from build123d import *

# Parameters (mm, degrees)
SKETCH1_W           = 74
SKETCH1_H           = 50
BOSS_EXTRUDE1_DEPTH = 10
SKETCH2_W           = 10
SKETCH2_H           = 50
BOSS_EXTRUDE2_DEPTH = 65
SKETCH3_R           = 5
CUT_EXTRUDE1_DEPTH  = 60
SKETCH4_R           = 5
CUT_EXTRUDE3_DEPTH  = 60


with BuildPart() as part:
    # Sketch1 → Boss-Extrude1 (new body)
    with BuildSketch(Plane(origin=(0, 0, 0), x_dir=(1, 0, 0), z_dir=(0, 1, 0))):
        Rectangle(SKETCH1_W, SKETCH1_H)
    extrude(amount=BOSS_EXTRUDE1_DEPTH)

    # Sketch2 → Boss-Extrude2 (add)
    with BuildSketch(Plane(origin=(0, 10, 0), x_dir=(1, 0, 0), z_dir=(0, 1, 0))):
        with Locations((-32, 0)):
            Rectangle(SKETCH2_W, SKETCH2_H)
        with Locations((32, 0)):
            Rectangle(SKETCH2_W, SKETCH2_H)
    extrude(amount=BOSS_EXTRUDE2_DEPTH)

    # Sketch3 → Cut-Extrude1 (cut)
    with BuildSketch(Plane(origin=(-27, 0, 0), x_dir=(0, 0, -1), z_dir=(1, 0, 0))):
        with Locations((0, 65)):
            Circle(SKETCH3_R)
    extrude(amount=-CUT_EXTRUDE1_DEPTH, mode=Mode.SUBTRACT)

    # Sketch4 → Cut-Extrude3 (cut)
    with BuildSketch(Plane.ZY.offset(-27)):
        with Locations((0, 60)):
            Circle(SKETCH4_R)
    extrude(amount=-CUT_EXTRUDE3_DEPTH, mode=Mode.SUBTRACT)


solid = part.part
Geometry check sheet. Reference: the model listing, model coordinates, mm. A direction names the side the tool comes from. Round coordinates to 2 decimals unless told otherwise and drop trailing zeros. Loops run counter-clockwise (first coordinate to the right, second up) from the corner with the lowest first, then second, coordinate; pieces in that order, holes last. Notation, with made-up numbers: (4.5, 52.25) - (13.5, 52.25) arc R33 cw to (13.5, 84.25) - close; hole circle Ø6 at (75.5, 34.5). An arc over 180 degrees is marked (long way). One line per question, with ' | ' between items. Start each with the question number.
1. Cross-section at C-C on x = -29.5. Record the cut outline in (y, z), then the cut area to 3 significant figures.
2. Cross-section at A-A on y = 39.5. Record the cut outline in (x, z), then the cut area to 3 significant figures.
3. Scan lines: line 1 (X direction, y = 28.5, z = -18); line 2 (Y direction, x = 31.5, z = 0); line 3 (Y direction, x = 8, z = 0). Record each from-to range of solid material in increasing order. Write a range as [from, to].
4. Tool access check on faces 1 (the face through (-32, 69, -3)), 2 (the face through (27, 42, 0)), 3 (the face through (-2.9, 9.5, -25)). Record the directions out of +Z, -Z, +X, -X, +Y, -Y that give a thin tool (end or side, any length) a straight path to the whole face; none if there is none.
5. Depth check by flat-ended pin: pin 1 (9 mm diameter, centred on y = 65, z = 0, fed in from -X); pin 2 (12 mm diameter, centred on x = 10.5, z = -8, fed in from +Y). Enter the tip coordinate at first touch or a pass-through.
6. Cross-section at D-D on x = -10.5. Record the cut outline in (y, z), then the cut area to 3 significant figures.
7. Draft check along Y on faces 4 (the face through (32, 75, 0)), 5 (the face through (32, 64, 3)), 6 (the face through (-37, 37, 0)). Enter one of: released by +Y, released by -Y, zero draft, split by the parting line, or undercut.
8. Cross-section at B-B on z = 16. Record the cut outline in (x, y).
Taken from the geometry:
1) outline: (0, -25) - (75, -25) - (75, 25) - (0, 25) - close; hole circle Ø10 at (65, 0) | area: 3,670 mm²
2) outline: (-37, -25) - (-27, -25) - (-27, 25) - (-37, 25) - close; (27, -25) - (37, -25) - (37, 25) - (27, 25) - close | area: 1,000 mm²
3) line 1: [-37, -27], [27, 37] | line 2: [0, 55], [65, 75] | line 3: [0, 10]
4) face 1: -X | face 2: +Z, -Z, +Y | face 3: -Z, +X, -X, +Y, -Y
5) pin 1: x = 27 | pin 2: y = 10
6) outline: (0, -25) - (10, -25) - (10, 25) - (0, 25) - close | area: 500 mm²
7) face 4: released by +Y | face 5: undercut | face 6: zero draft
8) outline: (-37, 0) - (37, 0) - (37, 75) - (27, 75) - (27, 10) - (-27, 10) - (-27, 75) - (-37, 75) - close
